from build123d import *

# Parameters (mm, degrees)
ESQUISSE1_W        = 170
ESQUISSE1_H        = 220
ESQUISSE1_R        = 11
ESQUISSE1_R_2      = 1.7
ESQUISSE1_R_3      = 1.5
ESQUISSE1_R_4      = 12
ESQUISSE1_R_5      = 5.5
ESQUISSE1_R_6      = 6.75
ESQUISSE1_W_2      = 21
ESQUISSE1_H_2      = 27.5
BOSS_EXTRU_1_DEPTH = 3


with BuildPart() as part:
    # Esquisse1 → Boss.-Extru.1 (new body)
    with BuildSketch(Plane.XY):
        with Locations((14.874803656, -69.780147352)):
            Rectangle(ESQUISSE1_W, ESQUISSE1_H)
        with Locations((-25.125196344, -69.780147352)):
            Circle(ESQUISSE1_R, mode=Mode.SUBTRACT)
        with Locations((-5.125196344, -89.780147352)):
            Circle(ESQUISSE1_R_2, mode=Mode.SUBTRACT)
        with Locations((-45.125196344, -89.780147352)):
            Circle(ESQUISSE1_R_2, mode=Mode.SUBTRACT)
        with Locations((-45.125196344, -49.780147352)):
            Circle(ESQUISSE1_R_2, mode=Mode.SUBTRACT)
        with Locations((-5.125196344, -49.780147352)):
            Circle(ESQUISSE1_R_2, mode=Mode.SUBTRACT)
        with Locations((83.874803656, -174.780147352)):
            Circle(ESQUISSE1_R_3, mode=Mode.SUBTRACT)
        with Locations((73.874803656, -174.780147352)):
            Circle(ESQUISSE1_R_3, mode=Mode.SUBTRACT)
        with Locations((83.874803656, 35.219852648)):
            Circle(ESQUISSE1_R_3, mode=Mode.SUBTRACT)
        with Locations((73.874803656, 35.219852648)):
            Circle(ESQUISSE1_R_3, mode=Mode.SUBTRACT)
        with Locations((-44.125196344, -174.780147352)):
            Circle(ESQUISSE1_R_3, mode=Mode.SUBTRACT)
        with Locations((-54.125196344, -174.780147352)):
            Circle(ESQUISSE1_R_3, mode=Mode.SUBTRACT)
        with Locations((-44.125196344, 35.219852648)):
            Circle(ESQUISSE1_R_3, mode=Mode.SUBTRACT)
        with Locations((-54.125196344, 35.219852648)):
            Circle(ESQUISSE1_R_3, mode=Mode.SUBTRACT)
        with Locations((39.874803656, 5.219852648)):
            Circle(ESQUISSE1_R_4, mode=Mode.SUBTRACT)
        with Locations((39.874803656, -41.030147352)):
            Circle(ESQUISSE1_R_5, mode=Mode.SUBTRACT)
        with Locations((39.874803656, -98.530147352)):
            Circle(ESQUISSE1_R_5, mode=Mode.SUBTRACT)
        with Locations((39.874803656, -151.105010126)):
            Circle(ESQUISSE1_R_6, mode=Mode.SUBTRACT)
        with Locations((18.874803656, -151.105010126)):
            Circle(ESQUISSE1_R_6, mode=Mode.SUBTRACT)
        with Locations((39.874803656, -69.780147352)):
            Rectangle(ESQUISSE1_W_2, ESQUISSE1_H_2, mode=Mode.SUBTRACT)
    extrude(amount=BOSS_EXTRU_1_DEPTH)


solid = part.part
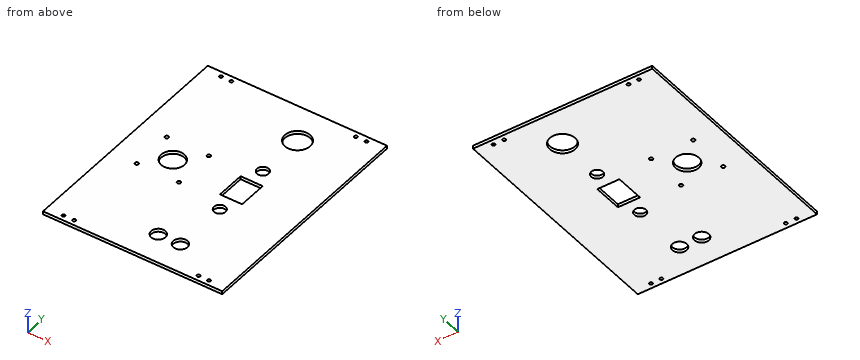
Source: CAD feature listing. Evaluate the final solid. Frame: model axes, mm. Round coordinates to 2 decimals unless told otherwise and drop trailing zeros. Order: outer loops, then holes, each group sorted by start corner. A loop starts at its lowest first (then second) coordinate and runs counter-clockwise, first axis right, second up. Notation, with made-up numbers: (29, 58.5) - (77, 58.5) arc R23 cw to (77, 97.5) - close; hole circle Ø4 at (40, 84). An arc over 180 degrees is marked (long way). Use a Markdown table: item, result. Add a question column.
1. Section query A-A (y = 10.5). Return the cut outline in (x, z), then the cut area to 3 significant figures.
2. Section query B-B (x = 17.5). Return the cut outline in (y, z), then the cut area to 3 significant figures.
3. Section query C-C (y = -73.5). Return the cut outline in (x, z).
4. Section query D-D (z = 2.25). Give the number of separate pieces and of enclosed holes in the cut face, then the cut area to 3 significant figures.
5. Line query: probe 1 along X at (y, z) = (-145, 1.3); probe 2 along Y at (x, z) = (22.5, 2.4); probe 3 along X at (y, z) = (-44.5, 1.85). Output: solid intervals per line, ascending.
Derived:
| question | item | result |
|---|---|---|
| 1 | outline | (-70.13, 0) - (29.1, 0) - (29.1, 3) - (-70.13, 3) - close; (50.65, 0) - (99.87, 0) - (99.87, 3) - (50.65, 3) - close |
| 1 | area | 445 mm2 |
| 2 | outline | (-179.78, 0) - (-157.71, 0) - (-157.71, 3) - (-179.78, 3) - close; (-144.5, 0) - (40.22, 0) - (40.22, 3) - (-144.5, 3) - close |
| 2 | area | 620 mm2 |
| 3 | outline | (-70.13, 0) - (-35.48, 0) - (-35.48, 3) - (-70.13, 3) - close; (-14.77, 0) - (29.37, 0) - (29.37, 3) - (-14.77, 3) - close; (50.37, 0) - (99.87, 0) - (99.87, 3) - (50.37, 3) - close |
| 4 | separate pieces | 1 |
| 4 | enclosed holes | 19 |
| 4 | area | 35,400 mm2 |
| 5 | probe 1 | -70.13 to 16, 21.75 to 37, 42.75 to 99.87 |
| 5 | probe 2 | -179.78 to -156.8, -145.41 to 40.22 |
| 5 | probe 3 | -70.13 to 35.61, 44.14 to 99.87 |
